Design review of the part shown in the three views and the two pictorial views. Dimensions are in mm from the part's minimum x, y and z. A direction names the side the tool comes from. Coordinates: 2 decimals unless noted, no trailing zeros. Loops run counter-clockwise (first coordinate to the right, second up) from the corner with the lowest first, then second, coordinate; pieces in that order, holes last. Notation, with made-up numbers: M 7.5,30 L 48.5,30 A17 cw 48.5,63 Z; hole C -36,42.5 d11. An arc over 180 degrees is marked long. Put each result on its own line as item: value. Start each with the question number.
(1) Take a section at D-D, the plane z = 38. Give the boundary of the cut face in (x, y), then the cut area to 3 significant figures.
(2) Clearance check with flat-ended pins moving along their axes: pin 1 (10 mm diameter, centred on x = 15, z = 70.5, fed in from +Y); pin 2 (1 mm diameter, centred on x = 30.5, z = 43.5, fed in from +Y); pin 3 (1.5 mm diameter, centred on x = 51, y = 19.5, fed in from +Z) (1 decimal). State where each tip first meets the part, or that it passes through.
(3) Take a section at B-B, the plane y = 21.5. Give the boundary of the cut face in (x, z) (1 decimal), then the cut area to 3 significant figures.
(4) For the marked faces 1 and 2, list the 3-axis set-ups (+Z, -Z, +X, -X, +Y, -Y) from which the entire face can be reached by the end or side of a thin tool; tool diameter is ignored.
(5) For probe 1 along Z at (x, y) = (19, 6) (1 decimal); probe 2 along Y at (x, z) = (31.5, 30.5), list the stretches that pass through material, from the lowest coordinate up. Write a range as [from, to].
(6) Take a section at C-C, the plane x = 19.5. Give the boundary of the cut face in (y, z) (1 decimal), then the cut area to 4 significant figures.
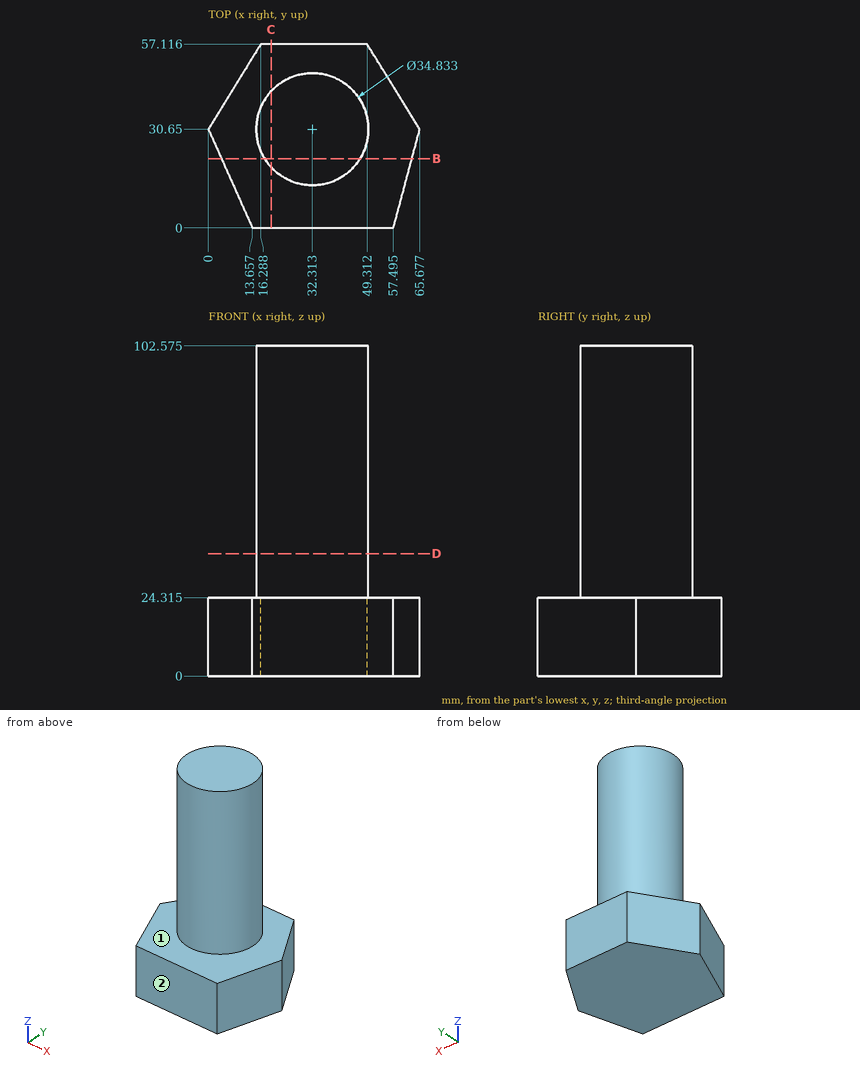
Computed values:
1. outline: C 32.31,30.65 d34.83
1. area: 953 mm^2
2. pin 1: stops at y = 42.97
2. pin 2: stops at y = 48.02
2. pin 3: stops at z = 24.3
3. outline: M 4.1,0 L 63.2,0 L 63.2,24.3 L 47.1,24.3 L 47.1,102.6 L 17.5,102.6 L 17.5,24.3 L 4.1,24.3 Z
3. area: 3,760 mm^2
4. face 1: +Z
4. face 2: +Z, -Z, +X, -X, -Y
5. probe 1: z = [0, 24.3]
5. probe 2: y = [13.25, 48.05]
6. outline: M 0,0 L 57.1,0 L 57.1,24.3 L 42.4,24.3 L 42.4,102.6 L 18.9,102.6 L 18.9,24.3 L 0,24.3 Z
6. area: 3,235 mm^2
